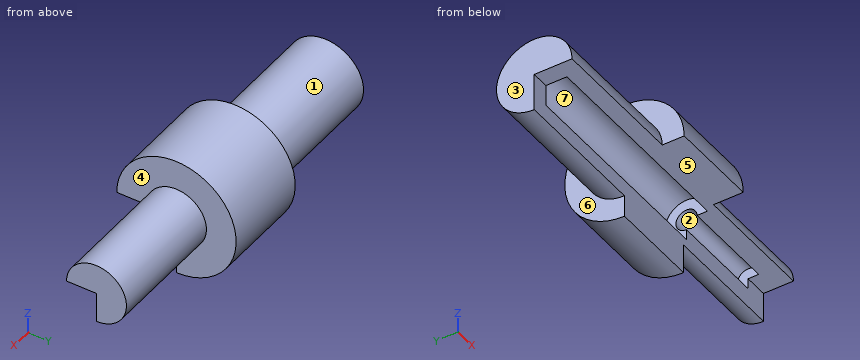
```python
from build123d import *

# Parameters (mm, degrees)
REVOLVE4_ANGLE = 270


with BuildPart() as part:
    # Sketch1 → Revolve4 (revolve)
    with BuildSketch(Plane(origin=(0, 0, 0), x_dir=(1, 0, 0), z_dir=(0, 1, 0))):
        Polygon((0, 32.550341736), (0, 0), (15.19362108, 0), (15.19362108, 18.201077386), (199.080833898, 18.201077386), (199.080833898, 9.100538693), (279.725137873, 9.100538693), (279.725137873, 0), (299.890300867, 0), (299.890300867, 25.830271184), (195.302050415, 25.830271184), (195.302050415, 51.450540163), (118.021239068, 51.450540163), (118.021239068, 32.550341736), align=None)
    revolve(axis=Axis((0, 0, 0), (1, 0, 0)), revolution_arc=REVOLVE4_ANGLE)


solid = part.part
```
Could you check a few things on this model? Use its own coordinates, in mm. Face numbers are marked on the shaded views. A direction names the side the tool comes from. Coordinates: 2 decimals unless noted, no trailing zeros. Order: outer loops, then holes, each group sorted by start corner. A loop starts at its lowest first (then second) coordinate and runs counter-clockwise, first axis right, second up. Notation, with made-up numbers: M 15.5,-12 L 45.5,-12 A27 cw 45.5,24 Z; hole C -39,82.25 d6. An arc over 180 degrees is marked long. Use a Markdown table: item, result. Add a question column.
Q1. I want a section at B-B on x = 214. List the corners of the cut face in (y, z) for me, then the cut area to 3 significant figures.
Q2. I want a section at C-C on y = -29.5. List the corners of the cut face in (x, z) for me, then the cut area to 3 significant figures.
Q3. I want a section at A-A on z = 14.5. List the corners of the cut face in (x, y) for me, then the cut area to 3 significant figures.
Q4. I'm going to push flat-ended pins straight in: pin 1 (15.5 mm diameter, centred on x = 83, y = -14.5, fed in from -Z); pin 2 (8 mm diameter, centred on x = 100, y = -38.5, fed in from -Z); pin 3 (1.5 mm diameter, centred on x = 144, z = -6.5, fed in from +Y); pin 4 (1.5 mm diameter, centred on x = 61, y = 15.5, fed in from -Z). Where does each tip first touch, or does it pass through?
Q5. If I drill on L1, parallel to X at y = 6, z = 40; L2, parallel to X at y = 11, z = -25.5; L3, parallel to Y at x = 21, z = 13, over which ranges is the centre line in solid material (lowest first)?
Q6. We'd pull the mould along Y, two halves only. Please class the marked faces 1, 2 and 3: pulls with the +Y half, pulls with the -Y half, needs draft (parallel to the pull), parting line crosses it, or undercut.
Q7. Which directions (+Z, -Z, +X, -X, +Y, -Y) give clear straight access to the entire face, cutting with the end or side of a thin tool? Please do the marked faces 4, 5, 6 and 7.
Q8. I want a section at D-D on x = 103. List the corners of the cut face in (y, z) for me, then the cut area to 3 significant figures.
Checked values:
| question | item | result |
|---|---|---|
| 1 | outline | M -25.83,0 L -9.1,0 A9.1 cw long 0,-9.1 L 0,-25.83 A25.83 ccw long Z |
| 1 | area | 1,380 mm² |
| 2 | outline | M 0,0 L 195.3,0 L 195.3,42.15 L 118.02,42.15 L 118.02,13.76 L 0,13.76 Z |
| 2 | area | 4,880 mm² |
| 3 | outline | M 0,-29.14 L 118.02,-29.14 L 118.02,-49.37 L 195.3,-49.37 L 195.3,-21.38 L 299.89,-21.38 L 299.89,21.38 L 195.3,21.38 L 195.3,49.37 L 118.02,49.37 L 118.02,29.14 L 0,29.14 Z; hole M 15.19,-11 L 199.08,-11 L 199.08,11 L 15.19,11 Z |
| 3 | area | 14,900 mm² |
| 4 | pin 1 | z = 0 |
| 4 | pin 2 | through |
| 4 | pin 3 | y = 51.13 |
| 4 | pin 4 | z = -29.02 |
| 5 | L1 | 118.02 to 195.3 |
| 5 | L2 | 0 to 195.3 |
| 5 | L3 | -29.84 to -12.74, 12.74 to 29.84 |
| 6 | face 1 | parting line crosses it |
| 6 | face 2 | undercut |
| 6 | face 3 | needs draft |
| 7 | face 4 | +X |
| 7 | face 5 | -Z, +X, -X, -Y |
| 7 | face 6 | -X |
| 7 | face 7 | none |
| 8 | outline | M -32.55,0 L -18.2,0 A18.2 cw long 0,-18.2 L 0,-32.55 A32.55 ccw long Z |
| 8 | area | 1,720 mm² |
